Source: three-view drawing plus pictorial views. Frame: mm from the lowest corner of the part. Round coordinates to 2 decimals unless told otherwise and drop trailing zeros. Order: outer loops, then holes, each group sorted by start corner. A loop starts at its lowest first (then second) coordinate and runs counter-clockwise, first axis right, second up. Notation, with made-up numbers: (72, 19) - (129, 19) arc R9 ccw to (129, 34) - close; hole circle Ø1 at (35.25, 58.25). An arc over 180 degrees is marked (long way). Use one line per item in the form item = value. Start each with the question number.
Q1. Cut plane D-D, the plane y = 1.15. Return the cut outline in (x, z).
Q2. Cut plane B-B, the plane x = 18. Return the cut outline in (y, z).
Q3. Draft query along X for the marked faces 1, 2, 3 and 4. Return one class per face: released by +X, released by -X, zero draft, split by the parting line, or undercut.
Q4. Ray query, line 1 (Z direction, x = 58, y = 1.75); line 2 (X direction, y = 3.95, z = 9.5); line 3 (X direction, y = 0.6, z = 3.25). Return the intervals inside material, ascending. Write a range as [from, to].
Q5. Pin query (flat end, axial travel): pin 1 Ø1.5 at (x, y) = (36, 4.5) entering from -Z; pin 2 Ø5 at (x, z) = (68, 2.5) entering from +Y. Return the tip coordinate at first contact, or that it passes through.
Q6. Cut plane C-C, the plane y = 4.05. Return the cut outline in (x, z), and give its area (3 significant figures).
Q7. Cut plane A-A, the plane z = 5. Return the cut outline in (x, y).
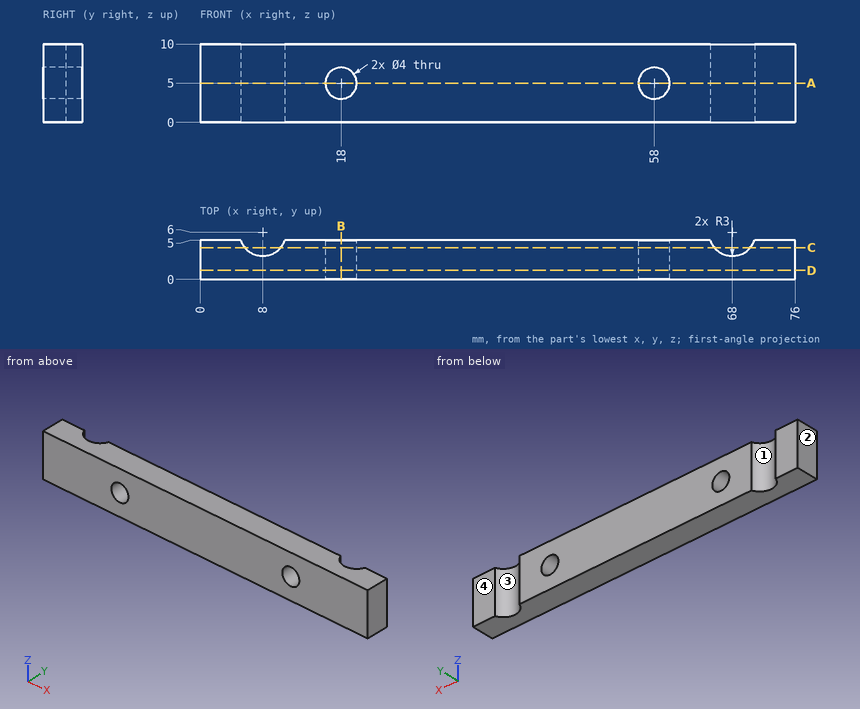
Completed:
q1.outline = (0, 0) - (76, 0) - (76, 10) - (0, 10) - close; hole circle Ø4 at (18, 5); hole circle Ø4 at (58, 5)
q2.outline = (0, 0) - (5, 0) - (5, 3) - (0, 3) - close; (0, 7) - (5, 7) - (5, 10) - (0, 10) - close
q3.face_1 = undercut
q3.face_2 = released by -X
q3.face_3 = undercut
q3.face_4 = zero draft
q4.line_1 = [0, 3], [7, 10]
q4.line_2 = [0, 5.81], [10.19, 65.81], [70.19, 76]
q4.line_3 = [0, 17.03], [18.97, 57.03], [58.97, 76]
q5.pin_1 = 0
q5.pin_2 = 4.34
q6.outline = (0, 0) - (5.72, 0) - (5.72, 10) - (0, 10) - close; (10.28, 0) - (65.72, 0) - (65.72, 10) - (10.28, 10) - close; (70.28, 0) - (76, 0) - (76, 10) - (70.28, 10) - close; hole circle Ø4 at (18, 5); hole circle Ø4 at (58, 5)
q6.area = 644 mm2
q7.outline = (0, 0) - (16, 0) - (16, 5) - (10.83, 5) arc R3 cw to (5.17, 5) - (0, 5) - close; (20, 0) - (56, 0) - (56, 5) - (20, 5) - close; (60, 0) - (76, 0) - (76, 5) - (70.83, 5) arc R3 cw to (65.17, 5) - (60, 5) - close
